Geometry check sheet. Reference: the model listing, model coordinates, mm. Face numbers are marked on the shaded views. A direction names the side the tool comes from. Coordinates: 2 decimals unless noted, no trailing zeros. Order: outer loops, then holes, each group sorted by start corner. A loop starts at its lowest first (then second) coordinate and runs counter-clockwise, first axis right, second up. Notation, with made-up numbers: M 47.5,-19.75 L 64.5,-19.75 A6 ccw 64.5,-9.75 Z; hole C 15.5,13 d1. An arc over 180 degrees is marked long. Use CSV: the item, a comma, the result in double quotes. Start each with the question number.
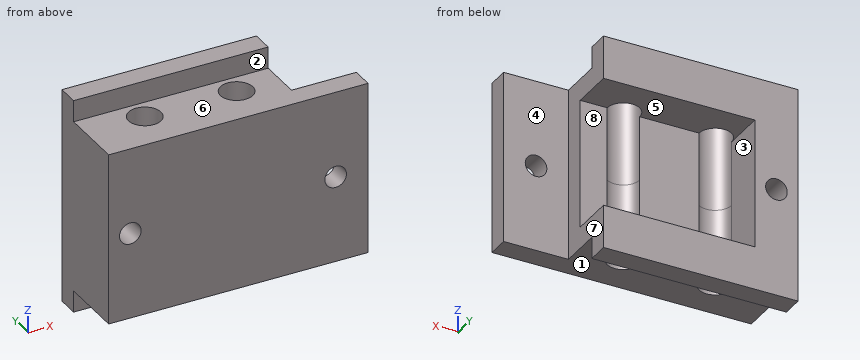
```python
from build123d import *

# Parameters (mm, degrees)
SKETCH1_W               = 76.2
SKETCH1_H               = 50.8
BOSS_EXTRUDE1_DEPTH     = 6.35
SKETCH2_W               = 57.15
SKETCH2_H               = 50.8
BOSS_EXTRUDE2_DEPTH     = 6.35
BOSS_EXTRUDE3_DEPTH     = 6.35
BOSS_EXTRUDE4_DEPTH     = 6.35
SKETCH5_R               = 3.175
CUT_EXTRUDE1_DEPTH      = 26.4
SKETCH6_R               = 4.7625
CUT_EXTRUDE2_DEPTH      = 32.75
CUT_EXTRUDE2_DEPTH_BACK = 32.75


with BuildPart() as part:
    # Sketch1 → Boss-Extrude1 (new body)
    with BuildSketch(Plane(origin=(0, 0, 0), x_dir=(1, 0, 0), z_dir=(0, 1, 0))):
        Rectangle(SKETCH1_W, SKETCH1_H)
    extrude(amount=BOSS_EXTRUDE1_DEPTH)

    # Sketch2 → Boss-Extrude2 (add)
    with BuildSketch(Plane(origin=(0, 6.35, 0), x_dir=(1, 0, 0), z_dir=(0, 1, 0))):
        with Locations((-9.525, 0)):
            Rectangle(SKETCH2_W, SKETCH2_H)
    extrude(amount=BOSS_EXTRUDE2_DEPTH)

    # Sketch3 → Boss-Extrude3 (add)
    with BuildSketch(Plane(origin=(0, 12.7, 0), x_dir=(1, 0, 0), z_dir=(0, 1, 0))):
        Polygon((19.05, 25.4), (-38.1, 25.4), (-38.1, -25.4), (19.05, -25.4), (19.05, -19.05), (-25.4, -19.05), (-25.4, 19.05), (19.05, 19.05), align=None)
    extrude(amount=BOSS_EXTRUDE3_DEPTH)

    # Sketch4 → Boss-Extrude4 (add)
    with BuildSketch(Plane(origin=(0, 19.05, 0), x_dir=(1, 0, 0), z_dir=(0, 1, 0))):
        Polygon((19.05, 19.05), (19.05, 31.75), (-38.1, 31.75), (-38.1, -31.75), (19.05, -31.75), (19.05, -19.05), (-25.4, -19.05), (-25.4, 19.05), align=None)
    extrude(amount=BOSS_EXTRUDE4_DEPTH)

    # Sketch5 → Cut-Extrude1 (cut, through all)
    with BuildSketch(Plane(origin=(0, 0, 0), x_dir=(1, 0, 0), z_dir=(0, 1, 0))):
        with Locations((-31.75, 0)):
            Circle(SKETCH5_R)
        with Locations((28.575, 0)):
            Circle(SKETCH5_R)
    extrude(amount=CUT_EXTRUDE1_DEPTH, mode=Mode.SUBTRACT)

    # Sketch6 → Cut-Extrude2 (cut, two sides)
    with BuildSketch(Plane.XY) as cut_extrude2_sk:
        with Locations((-20.6375, 12.7)):
            Circle(SKETCH6_R)
        with Locations((6.35, 12.7)):
            Circle(SKETCH6_R)
    extrude(amount=CUT_EXTRUDE2_DEPTH, mode=Mode.SUBTRACT)
    extrude(cut_extrude2_sk.sketch, amount=-CUT_EXTRUDE2_DEPTH_BACK, mode=Mode.SUBTRACT)


solid = part.part
```
1) Section check B-B on y = 14.75. Record the boundary of the cut face in (x, z) (3 decimals).
2) Set-up check for the marked faces 1, 2, 3 and 4: record each of +Z, -Z, +X, -X, +Y, -Y from which the full face is reachable in a straight line by a thin tool's end or side.
3) Gauge pin test, flat ends, axial feed: P1, Ø8.5, axis at x = -20.64, y = 12.7, coming from the +Z side; P2, Ø15, axis at x = 9.5, y = 5.5, coming from the -Z side; P3, Ø5, axis at x = -1.5, z = -28, coming from the -Y side; P4, Ø6.5, axis at y = 19, z = -5.5, coming from the +X side. Record the tip position at first contact, or that the pin passes through.
4) Section check C-C on x = -31.75. Record the boundary of the cut face in (y, z) (3 decimals).
5) Material ranges on line 1 along X through (y, z) = (3.5, 0) (3 decimals); line 2 along Z through (x, y) = (-10, 22.75); line 3 along Z through (x, y) = (15.5, 1), recorded low to high.
6) Draft check along Z on the marked faces 5, 6, 7 and 8. Enter one of: +Z half, -Z half, draft (parallel to the pull), parting line (faces both ways), or undercut.
7) Section check A-A on z = -24. State how many separate pieces and enclosed holes the cut face has, then the cut area to 3 significant figures.
8) Section check D-D on y = 9. Record the boundary of the cut face in (x, z) (3 decimals), then the cut area to 3 significant figures.
Results are:
1,outline,"M -38.1,-25.4 L -24.936,-25.4 L -24.936,-19.05 L -25.4,-19.05 L -25.4,19.05 L -24.936,19.05 L -24.936,25.4 L -38.1,25.4 Z; M -16.339,-25.4 L 2.051,-25.4 L 2.051,-19.05 L -16.339,-19.05 Z; M -16.339,19.05 L 2.051,19.05 L 2.051,25.4 L -16.339,25.4 Z; M 10.649,-25.4 L 19.05,-25.4 L 19.05,-19.05 L 10.649,-19.05 Z; M 10.649,19.05 L 19.05,19.05 L 19.05,25.4 L 10.649,25.4 Z; hole C -31.75,0 d6.35"
2,face 1,"-Z, +X, -X, -Y"
2,face 2,"+Z, +X, -X, -Y"
2,face 3,"+X, +Y"
2,face 4,"+Z, -Z, +X, +Y"
3,P1,"passes through"
3,P2,"stops at z = -25.4"
3,P3,"stops at y = 19.05"
3,P4,"stops at x = -25.4"
4,outline,"M 0,-25.4 L 19.05,-25.4 L 19.05,-31.75 L 25.4,-31.75 L 25.4,-3.175 L 0,-3.175 Z; M 0,3.175 L 25.4,3.175 L 25.4,31.75 L 19.05,31.75 L 19.05,25.4 L 0,25.4 Z"
5,line 1,"x = -38.1 to -34.925, -28.575 to 25.4, 31.75 to 38.1"
5,line 2,"z = -31.75 to -19.05, 19.05 to 31.75"
5,line 3,"z = -25.4 to 25.4"
6,face 5,"undercut"
6,face 6,"+Z half"
6,face 7,"draft"
6,face 8,"undercut"
7,separate pieces,"1"
7,enclosed holes,"2"
7,area,"1,430 mm²"
8,outline,"M -38.1,-25.4 L -23.636,-25.4 L -23.636,25.4 L -38.1,25.4 Z; M -17.639,-25.4 L 3.351,-25.4 L 3.351,25.4 L -17.639,25.4 Z; M 9.349,-25.4 L 19.05,-25.4 L 19.05,25.4 L 9.349,25.4 Z; hole C -31.75,0 d6.35"
8,area,"2,260 mm²"
